Geometry: final body of the model. Coordinates: model frame, mm. Face numbers are marked on the shaded views. A direction names the side the tool comes from. Coordinates: 2 decimals unless noted, no trailing zeros. Write each loop counter-clockwise with the first axis right and the second up, starting at its lowest first coordinate (ties: lowest second). Pieces come first, ordered by that corner, then holes. Notation, with made-up numbers: M 80,-19.75 L 135,-19.75 A12 cw 135,3.25 Z; hole C 54,24 d2. An arc over 180 degrees is marked long. Write item = value, one per line. Start each with the question number.
Item 1: Ray query, L1, parallel to X at y = 62.55, z = 0 (3 decimals); L2, parallel to X at y = 83, z = 0; L3, parallel to Z at x = -14, y = 64. Return the intervals inside material, ascending. Write a range as [from, to].
Item 2: First-contact query: pin 1 Ø8 at (x, y) = (-9.5, 66) entering from -Z; pin 2 Ø1.8 at (x, z) = (-14.5, 0) entering from -Y; pin 3 Ø4 at (y, z) = (61, -12.5) entering from +X. Flat tips, straight axial feed; report the tip coordinate or a pass-through.
Item 3: Section B-B on y = 2. Output: boundary loops of the cut face in (x, z) (3 decimals).
Item 4: Section A-A on y = 30. Output: boundary loops of the cut face in (x, z) (3 decimals).
Item 5: Reachability of the marked faces 1, 2 and 3 from +Z, -Z, +X, -X, +Y, -Y: full face, straight path, thin tool, end or side. Return the list, or none.
from build123d import *

# Parameters (mm, degrees)
SKETCH1_R           = 21.125
BOSS_EXTRUDE1_DEPTH = 66.5
SKETCH2_R           = 7.2
BOSS_EXTRUDE2_DEPTH = 4
SKETCH3_R           = 2.5
BOSS_EXTRUDE3_DEPTH = 6.2
SKETCH4_R           = 8.7
BOSS_EXTRUDE4_DEPTH = 4.8
BOSS_EXTRUDE5_START = 16.4
SKETCH5_R           = 2.5
BOSS_EXTRUDE5_DEPTH = 16.4
SKETCH6_R           = 1.5
CUT_EXTRUDE1_DEPTH  = 5
BOSS_EXTRUDE6_START = -40
BOSS_EXTRUDE6_DEPTH = 40
CUT_EXTRUDE2_START  = -6
CUT_EXTRUDE2_DEPTH  = 6
FILLET1_R           = 2


with BuildPart() as part:
    # Sketch1 → Boss-Extrude1 (new body)
    with BuildSketch(Plane(origin=(0, 0, 0), x_dir=(1, 0, 0), z_dir=(0, 1, 0))):
        with Locations(Location((0, 0, 0), (0, 0, 270))):
            Circle(SKETCH1_R)
    extrude(amount=BOSS_EXTRUDE1_DEPTH)

    # Sketch2 → Boss-Extrude2 (add)
    with BuildSketch(Plane.XZ):
        with Locations(Location((0, 0, 0), (0, 0, 270))):
            Circle(SKETCH2_R)
    extrude(amount=BOSS_EXTRUDE2_DEPTH)

    # Sketch3 → Boss-Extrude3 (add)
    with BuildSketch(Plane.XZ.offset(4)):
        with Locations(Location((0, 0, 0), (0, 0, 90))):
            Circle(SKETCH3_R)
    extrude(amount=BOSS_EXTRUDE3_DEPTH)

    # Sketch4 → Boss-Extrude4 (add)
    with BuildSketch(Plane(origin=(0, 66.5, 0), x_dir=(1, 0, 0), z_dir=(0, 1, 0))):
        with Locations(Location((0, 0, 0), (0, 0, 270))):
            Circle(SKETCH4_R)
    extrude(amount=BOSS_EXTRUDE4_DEPTH)

    # Sketch5 → Boss-Extrude5 (add)
    with BuildSketch(Plane(origin=(0, 71.3, 0), x_dir=(1, 0, 0), z_dir=(0, 1, 0)).offset(BOSS_EXTRUDE5_START)):
        with Locations(Location((0, 0, 0), (0, 0, 270))):
            Circle(SKETCH5_R)
    extrude(amount=-BOSS_EXTRUDE5_DEPTH)

    # Sketch6 → Cut-Extrude1 (cut)
    with BuildSketch(Plane(origin=(0, 66.5, 0), x_dir=(1, 0, 0), z_dir=(0, 1, 0))):
        with Locations(Location((14.5, 0, 0), (0, 0, 270))):
            Circle(SKETCH6_R)
        with Locations(Location((-14.5, 0, 0), (0, 0, 270))):
            Circle(SKETCH6_R)
    extrude(amount=-CUT_EXTRUDE1_DEPTH, mode=Mode.SUBTRACT)

    # Sketch7 → Boss-Extrude6 (add)
    with BuildSketch(Plane(origin=(0, 66.5, 0), x_dir=(1, 0, 0), z_dir=(0, 1, 0)).offset(BOSS_EXTRUDE6_START)):
        with BuildLine():
            Line((1.25, 21.087985323), (1.25, 22.164780622))
            ThreePointArc((1.25, 22.164780622), (0, -22.2), (-1.25, 22.164780622))
            Line((-1.25, 22.164780622), (-1.25, 21.087985323))
            ThreePointArc((-1.25, 21.087985323), (0, -21.125), (1.25, 21.087985323))
        make_face()
    extrude(amount=BOSS_EXTRUDE6_DEPTH)

    # Sketch7<3> → Cut-Extrude2 (cut)
    with BuildSketch(Plane(origin=(0, 66.5, 0), x_dir=(1, 0, 0), z_dir=(0, 1, 0)).offset(CUT_EXTRUDE2_START)):
        with BuildLine():
            Line((1.25, 21.087985323), (1.25, 22.164780622))
            ThreePointArc((1.25, 22.164780622), (0, -22.2), (-1.25, 22.164780622))
            Line((-1.25, 22.164780622), (-1.25, 21.087985323))
            ThreePointArc((-1.25, 21.087985323), (0, -21.125), (1.25, 21.087985323))
        make_face()
    extrude(amount=CUT_EXTRUDE2_DEPTH, mode=Mode.SUBTRACT)

    # Fillet1
    fillet1_edges = [part.edges().sort_by_distance(p)[0] for p in [
        (1.25, 66.5, 21.087985323),
    ]]
    fillet(fillet1_edges, radius=FILLET1_R)


solid = part.part
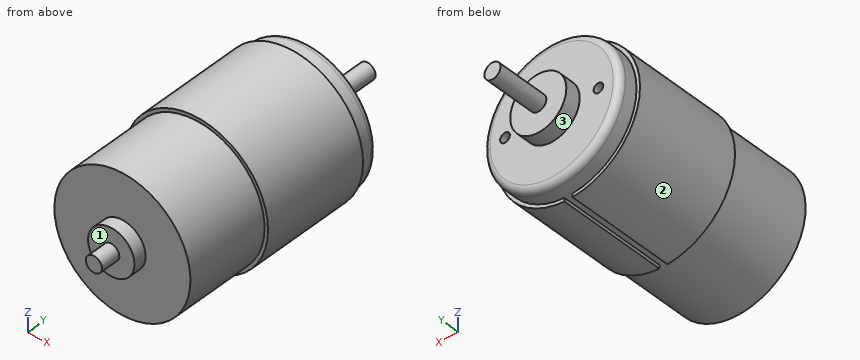
Responses:
q1.L1 = [-21.125, -16], [-13, 13], [16, 21.125]
q1.L2 = [-2.5, 2.5]
q1.L3 = [-15.82, -1.41], [1.41, 15.82]
q2.pin_1 = -20.33
q2.pin_2 = 0
q2.pin_3 = 19.53
q3.outline = C 0,0 d42.25
q4.outline = M -1.25,-22.165 L -1.25,-21.088 A21.125 ccw 1.25,-21.088 L 1.25,-22.165 A22.2 ccw long Z
q5.face_1 = -Y
q5.face_2 = +Y, -Y
q5.face_3 = +Y
